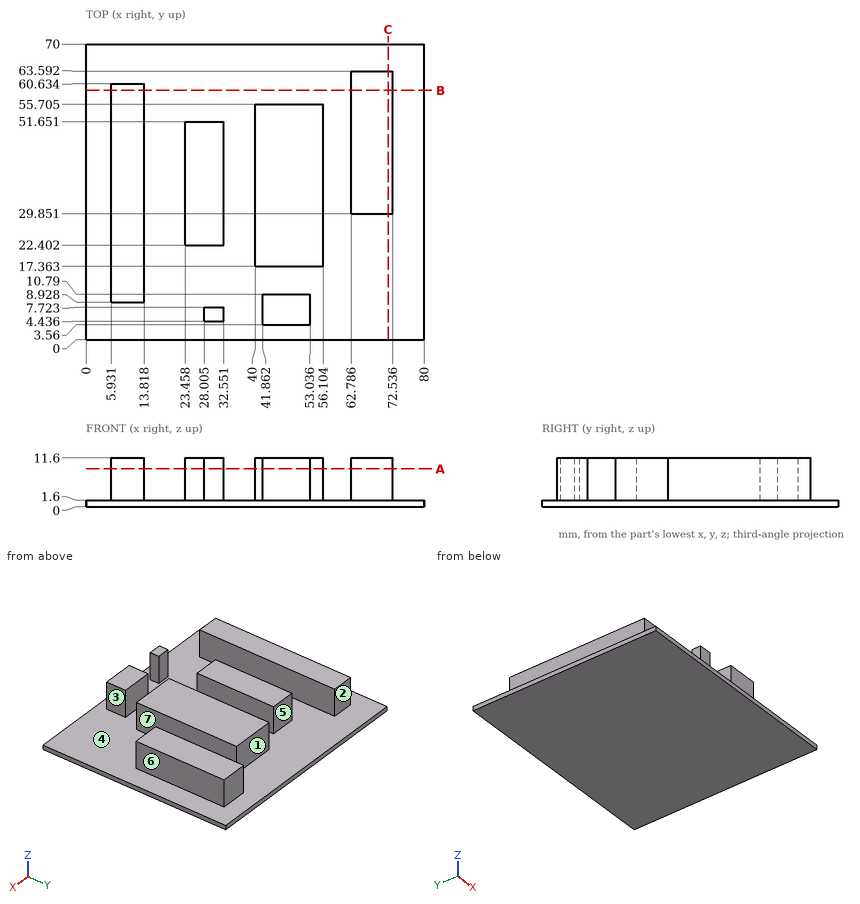
Can you work these out from the drawing? Everything is in mm from the part's minimum corner. A direction names the side the tool comes from. Give positions to 0.01 mm unless a question says otherwise; leave off trailing zeros. Write each loop counter-clockwise with the first axis right and the second up, starting at its lowest first coordinate (ties: lowest second). Pieces come first, ordered by that corner, then holes. Notation, with made-up numbers: (72, 65.25) -> (114, 65.25) arc R35 ccw to (114, 99.25) -> close; hole circle Ø10 at (54.25, -5). An arc over 180 degrees is marked (long way). Write each question's results on one line, items separated by ' | '. Start each with the question number.
Q1. Suppose I cut it at B-B, the plane y = 59. List the corners of the cut face in (x, z) for me (1 decimal).
Q2. Suppose I cut it at C-C, the plane x = 71.5. List the corners of the cut face in (y, z) for me.
Q3. Suppose I cut it at A-A, the plane z = 9. State how many separate pieces and enclosed holes the cut face has, and give its area (3 significant figures).
Q4. Which directions (+Z, -Z, +X, -X, +Y, -Y) give clear straight access to the entire face, cutting with the end or side of a thin tool? Please do the marked faces 5, 6 and 7.
Q5. I'm going to push flat-ended pins straight in: pin 1 Ø3 at (x, z) = (69, 6.5) entering from +Y; pin 2 Ø3 at (x, z) = (45, 6.5) entering from +Y (1 decimal); pin 3 Ø5 at (y, z) = (23, 4.5) entering from -X. Where does each tip first touch, or does it pass through?
Q6. We'd pull the mould along X, two halves only. Please class the marked faces 1, 2, 3 and 4: +X half, -X half, draft (parallel to the pull), parting line (faces both ways), or undercut.
Q7. I need wall thicknesses on probe 1 along X at (y, z) = (26, 6); probe 2 along Y at (x, z) = (49, 4) (1 decimal); probe 3 along X at (y, z) = (9, 6.5). Which ranges of each line are inside material? Lowest first, please.
Outcome:
1) outline: (0, 0) -> (80, 0) -> (80, 1.6) -> (72.5, 1.6) -> (72.5, 11.6) -> (62.8, 11.6) -> (62.8, 1.6) -> (13.8, 1.6) -> (13.8, 11.6) -> (5.9, 11.6) -> (5.9, 1.6) -> (0, 1.6) -> close
2) outline: (0, 0) -> (70, 0) -> (70, 1.6) -> (63.59, 1.6) -> (63.59, 11.6) -> (29.85, 11.6) -> (29.85, 1.6) -> (0, 1.6) -> close
3) separate pieces: 6 | enclosed holes: 0 | area: 1,720 mm2
4) face 5: +Z, +Y | face 6: +Z, +X, +Y, -Y | face 7: +Z, +Y, -Y
5) pin 1: y = 63.59 | pin 2: y = 55.7 | pin 3: x = 5.93
6) face 1: undercut | face 2: draft | face 3: +X half | face 4: undercut
7) probe 1: 5.93 to 13.82, 23.46 to 32.55, 40 to 56.1 | probe 2: 3.6 to 10.8, 17.4 to 55.7 | probe 3: 5.93 to 13.82, 41.86 to 53.04
